```python
from build123d import *

# Parameters (mm, degrees)
EXTRUDE_1_DEPTH = 2
SKETCH_2_R      = 1
EXTRUDE_2_DEPTH = 2
SKETCH_3_R      = 1
EXTRUDE_3_DEPTH = 2


with BuildPart() as part:
    # 草图1 → 凸台-拉伸1 (new body)
    with BuildSketch(Plane.XY):
        with BuildLine():
            Line((-16.391109626, -2), (33.608890374, -2))
            ThreePointArc((33.608890374, -2), (35.608890374, 0), (33.608890374, 2))
            Line((33.608890374, 2), (-16.391109626, 2))
            ThreePointArc((-16.391109626, 2), (-18.391109626, 0), (-16.391109626, -2))
        make_face()
    extrude(amount=EXTRUDE_1_DEPTH)

    # 草图2 → 凸台-拉伸2 (add)
    with BuildSketch(Plane.XY.offset(2)):
        with Locations((33.608890374, 0)):
            Circle(SKETCH_2_R)
    extrude(amount=EXTRUDE_2_DEPTH)

    # 草图3 → 凸台-拉伸3 (add)
    with BuildSketch(Plane(origin=(0, 0, 0), x_dir=(-1, 0, 0), z_dir=(0, 0, -1))):
        with Locations((16.391109626, 0)):
            Circle(SKETCH_3_R)
    extrude(amount=EXTRUDE_3_DEPTH)


solid = part.part
```
Check sheet for the modelled part. Datum: model origin and axes. Units: mm. A direction names the side the tool comes from. Give positions to 0.01 mm unless a question says otherwise; leave off trailing zeros. Write each loop counter-clockwise with the first axis right and the second up, starting at its lowest first coordinate (ties: lowest second). Pieces come first, ordered by that corner, then holes.
Item 1: Cross-section at A-A (y = -0.55). Enter the section's corners in (x, z).
Item 2: Cross-section at C-C (x = 31). Enter the section's corners in (y, z), and give its area (3 significant figures).
Item 3: Cross-section at D-D (z = 1.4). Enter the section's corners in (x, y), and give its area (3 significant figures).
Item 4: Cross-section at B-B (z = 3.35). Enter the section's corners in (x, y), and give its area (3 significant figures).
Item 5: Gauge pin test, flat ends, axial feed: pin 1 (2 mm diameter, centred on x = -6.5, y = 0, fed in from +Z); pin 2 (1.5 mm diameter, centred on y = 1.5, z = 2, fed in from +X); pin 3 (2 mm diameter, centred on x = 6.5, y = 0, fed in from -Z). Record the tip position at first contact, or that the pin passes through.
Item 6: Scan lines: L1, parallel to X at y = 0.15, z = 3.5; L2, parallel to Z at x = 0, y = -0.65; L3, parallel to X at y = -0.15, z = -0.4. Record each from-to range of solid material in increasing order.
Item 7: Draft check along Y on faces 1 (the face through (9, 2, 1)), 2 (the face through (35.61, -0.04, 0.99)), 3 (the face through (8, 0, 2)), 4 (the face through (8, -2, 1)). Enter one of: released by +Y, released by -Y, zero draft, split by the parting line, or undercut.
Item 8: Access from +Z, -Z, +X, -X, +Y, -Y to the whole of each face (thin tool, end or side, straight path). Record for faces 5 (the face through (34.563, 0.3, 2.986)), 6 (the face through (34, 0, 4)), 7 (the face through (-17.315, -0.383, -0.986)).
Report:
1. outline: (-18.31, 0) - (-17.23, 0) - (-17.23, -2) - (-15.56, -2) - (-15.56, 0) - (35.53, 0) - (35.53, 2) - (34.44, 2) - (34.44, 4) - (32.77, 4) - (32.77, 2) - (-18.31, 2) - close
2. outline: (-2, 0) - (2, 0) - (2, 2) - (-2, 2) - close
2. area: 8.00 mm2
3. outline: (-16.39, -2) - (33.61, -2) arc R2 ccw to (33.61, 2) - (-16.39, 2) arc R2 ccw to start
3. area: 213 mm2
4. outline: circle Ø2 at (33.61, 0)
4. area: 3.14 mm2
5. pin 1: stops at z = 2
5. pin 2: stops at x = 35.46
5. pin 3: stops at z = 0
6. L1: x = 32.62 to 34.6
6. L2: z = 0 to 2
6. L3: x = -17.38 to -15.4
7. face 1: released by +Y
7. face 2: split by the parting line
7. face 3: zero draft
7. face 4: released by -Y
8. face 5: +Z
8. face 6: +Z, +X, -X, +Y, -Y
8. face 7: -Z
